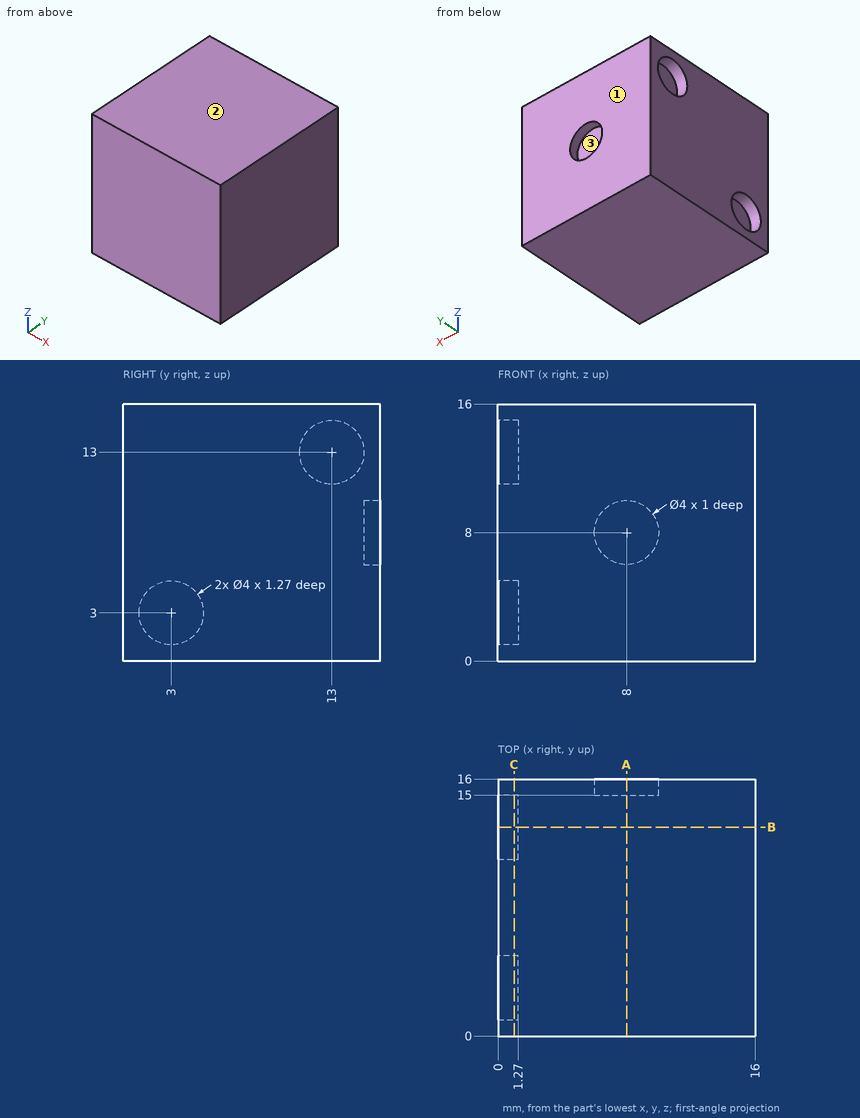
Geometry: see drawing. Coordinates: mm, zero at the bounding-box minimum. Give positions to 0.01 mm unless a question says otherwise; leave off trailing zeros. Loops run counter-clockwise (first coordinate to the right, second up) from the corner with the lowest first, then second, coordinate; pieces in that order, holes last. Notation, with made-up numbers: (36.25, 1) -> (68.25, 1) arc R28 ccw to (68.25, 30) -> close; hole circle Ø6 at (65, -13). An arc over 180 degrees is marked (long way). Put each result on its own line as item: value.
1. Pin query (flat end, axial travel): P1, Ø2, axis at y = 12.5, z = 13.5, coming from the -X side. Return the tip coordinate at first contact, or that it passes through.
Taken from the geometry:
P1: stops at x = 1.27
2. Cut plane C-C (x = 1). Return the cut outline in (y, z), plus the area to 3 significant figures.
Taken from the geometry:
outline: (0, 0) -> (16, 0) -> (16, 16) -> (0, 16) -> close; hole circle Ø4 at (3, 3); hole circle Ø4 at (13, 13)
area: 231 mm2
3. Cut plane B-B (y = 13). Return the cut outline in (x, z), plus the area to 3 significant figures.
Taken from the geometry:
outline: (0, 0) -> (16, 0) -> (16, 16) -> (0, 16) -> (0, 15) -> (1.27, 15) -> (1.27, 11) -> (0, 11) -> close
area: 251 mm2
4. Pull-direction query (Z, two-part tool) for the marked faces 1, 2 and 3; classes: released by +Z, released by -Z, zero draft, split by the parting line, or undercut.
Taken from the geometry:
face 1: zero draft
face 2: released by +Z
face 3: undercut
5. Cut plane A-A (x = 8). Return the cut outline in (y, z), plus the area to 3 significant figures.
Taken from the geometry:
outline: (0, 0) -> (16, 0) -> (16, 6) -> (15, 6) -> (15, 10) -> (16, 10) -> (16, 16) -> (0, 16) -> close
area: 252 mm2
6. Ray query, line 1 along Z through (x, y) = (0.4, 3); line 2 along Z through (x, y) = (0.65, 13); line 3 along X through (y, z) = (12.75, 11.25). Return the intervals inside material, ascending. Write a range as [from, to].
Taken from the geometry:
line 1: z = [0, 1], [5, 16]
line 2: z = [0, 11], [15, 16]
line 3: x = [1.27, 16]
